from build123d import *

# Parameters (mm, degrees)
SKETCH1_W           = 80.7
SKETCH1_H           = 20
SKETCH1_R           = 2.5
BOSS_EXTRUDE1_DEPTH = 10
FILLET1_R           = 10


with BuildPart() as part:
    # Sketch1 → Boss-Extrude1 (new body)
    with BuildSketch(Plane.XY):
        Rectangle(SKETCH1_W, SKETCH1_H)
        with Locations((-35.35, 0)):
            Circle(SKETCH1_R, mode=Mode.SUBTRACT)
        with Locations((35.35, 0)):
            Circle(SKETCH1_R, mode=Mode.SUBTRACT)
    extrude(amount=BOSS_EXTRUDE1_DEPTH)

    # Fillet1
    fillet1_edges = [part.edges().sort_by_distance(p)[0] for p in [
        (40.35, -10, 5),
        (40.35, 10, 5),
        (-40.35, -10, 5),
        (-40.35, 10, 5),
    ]]
    fillet(fillet1_edges, radius=FILLET1_R - 0.0001)  # a hair under: the kernel refuses the full size


solid = part.part
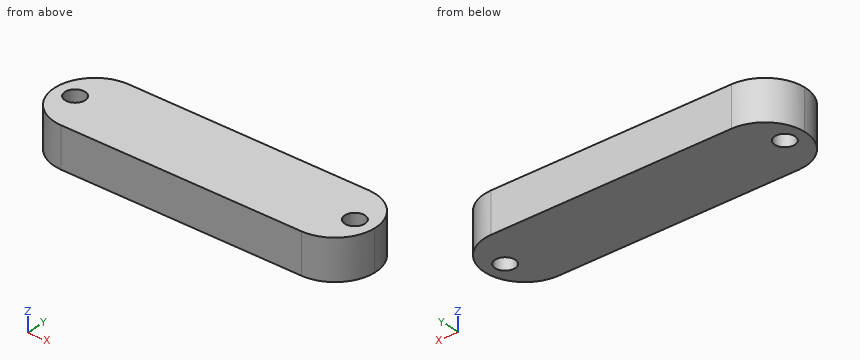
The listing builds one solid part. Answer for the finished solid, in the listing's coordinates (mm). Give positions to 0.01 mm unless a question says otherwise; leave off trailing zeros. Write each loop counter-clockwise with the first axis right and the second up, starting at its lowest first coordinate (ties: lowest second). Pieces come first, ordered by that corner, then holes.
Item 1: Flat-ended cylindrical pins translate along their axes: P1, Ø6, axis at y = 4.5, z = 2.5, coming from the -X side; P2, Ø5, axis at y = 7, z = 7.5, coming from the -X side. Find the tip coordinate at first contact, or state that the pin passes through.
Item 2: Find the intervals of material crossed by line 1 along X through (y, z) = (0.25, 1); line 2 along Y through (x, z) = (-35.35, 6); line 3 along X through (y, z) = (7.75, 3), in increasing order.
Item 3: Section C-C, the plane y = 3.5 is taken. Write down the section's boundary in (x, z), plus the area to 3 significant figures.
Item 4: Section B-B, the plane x = -35.35 is taken. Write down the section's boundary in (y, z), plus the area to 3 significant figures.
Item 5: Section A-A, the plane z = 7.75 is taken. Count the separate pieces of the cut face and the enclosed holes in it, plus the area to 3 significant figures.
Item 6: Section D-D, the plane y = 6.5 is taken. Write down the section's boundary in (x, z), plus the area to 3 significant figures.
Completed:
1. P1: stops at x = -40.24
1. P2: stops at x = -39.28
2. line 1: x = -40.35 to -37.84, -32.86 to 32.86, 37.84 to 40.35
2. line 2: y = -8.66 to -2.5, 2.5 to 8.66
2. line 3: x = -36.67 to 36.67
3. outline: (-39.72, 0) - (39.72, 0) - (39.72, 10) - (-39.72, 10) - close
3. area: 794 mm2
4. outline: (-8.66, 0) - (-2.5, 0) - (-2.5, 10) - (-8.66, 10) - close; (2.5, 0) - (8.66, 0) - (8.66, 10) - (2.5, 10) - close
4. area: 123 mm2
5. separate pieces: 1
5. enclosed holes: 2
5. area: 1,490 mm2
6. outline: (-37.95, 0) - (37.95, 0) - (37.95, 10) - (-37.95, 10) - close
6. area: 759 mm2
